The figure shows three views and two pictorial views of one solid part (mm, origin at its lowest corner). Answer the questions. Round coordinates to 2 decimals unless told otherwise and drop trailing zeros. Write each loop counter-clockwise with the first axis right and the second up, starting at its lowest first coordinate (ties: lowest second). Pieces come first, ordered by that corner, then holes. Notation, with made-up numbers: (64, 55.5) - (104, 55.5) arc R15 ccw to (104, 79.5) - close; hole circle Ø8 at (44, 49.5). An arc over 180 degrees is marked (long way). Answer as CSV lines item,"result". Start each with the question number.
Item 1: Flat-ended cylindrical pins translate along their axes: pin 1 (3.5 mm diameter, centred on x = 3.5, z = 65, fed in from +Y); pin 2 (1.4 mm diameter, centred on x = 3.5, z = 50, fed in from +Y). Find the tip coordinate at first contact, or state that the pin passes through.
Item 2: A cutting plane is placed at B-B on z = 50. Determine the outline of the cut face in (x, y).
Item 3: A cutting plane is placed at C-C on x = 3.5. State how many separate pieces and enclosed holes the cut face has, and give its area (3 significant figures).
Item 4: Straight lines are drawn through the part: line 1 along Z through (x, y) = (3.5, 2.2); line 2 along X through (y, z) = (4.2, 20); line 3 along X through (y, z) = (0.85, 65). For each, find the intervals that lie inside material, in ascending order. Write a range as [from, to].
Item 5: A cutting plane is placed at A-A on y = 0.75. Determine the outline of the cut face in (x, z).
Item 6: A cutting plane is placed at D-D on y = 4.1. Determine the outline of the cut face in (x, z), and give its area (3 significant figures).
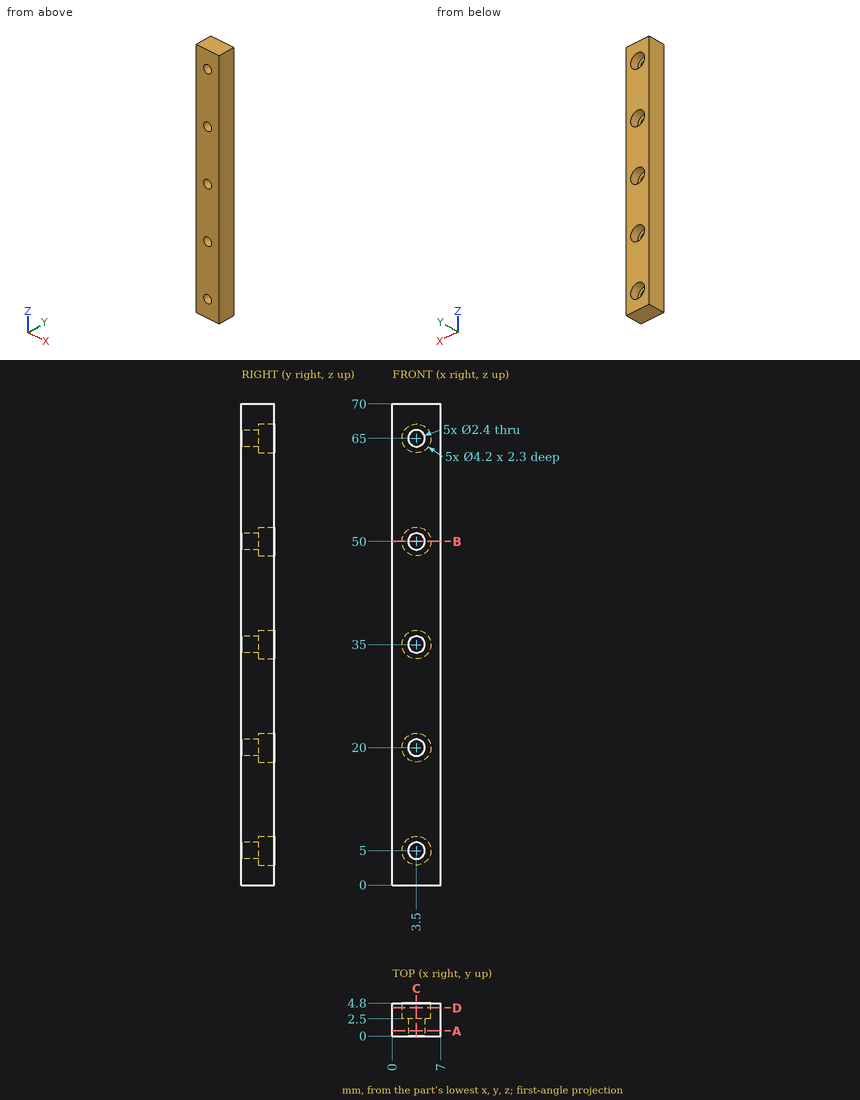
Geometry says:
1,pin 1,"stops at y = 2.5"
1,pin 2,"passes through"
2,outline,"(0, 0) - (2.3, 0) - (2.3, 2.5) - (1.4, 2.5) - (1.4, 4.8) - (0, 4.8) - close; (4.7, 0) - (7, 0) - (7, 4.8) - (5.6, 4.8) - (5.6, 2.5) - (4.7, 2.5) - close"
3,separate pieces,"6"
3,enclosed holes,"0"
3,area,"258 mm^2"
4,line 1,"z = [0, 3.8], [6.2, 18.8], [21.2, 33.8], [36.2, 48.8], [51.2, 63.8], [66.2, 70]"
4,line 2,"x = [0, 1.4], [5.6, 7]"
4,line 3,"x = [0, 2.3], [4.7, 7]"
5,outline,"(0, 0) - (7, 0) - (7, 70) - (0, 70) - close; hole circle Ø2.4 at (3.5, 5); hole circle Ø2.4 at (3.5, 20); hole circle Ø2.4 at (3.5, 35); hole circle Ø2.4 at (3.5, 50); hole circle Ø2.4 at (3.5, 65)"
6,outline,"(0, 0) - (7, 0) - (7, 70) - (0, 70) - close; hole circle Ø4.2 at (3.5, 5); hole circle Ø4.2 at (3.5, 20); hole circle Ø4.2 at (3.5, 35); hole circle Ø4.2 at (3.5, 50); hole circle Ø4.2 at (3.5, 65)"
6,area,"421 mm^2"
